from build123d import *

# Parameters (mm, degrees)
BOSS_EXTRUDE1_START = -169
SKETCH1_R           = 8
BOSS_EXTRUDE1_DEPTH = 294
SKETCH3_R           = 8
BOSS_EXTRUDE2_START = 159
SKETCH4_W           = 5.5
SKETCH4_H           = 3
BOSS_EXTRUDE2_DEPTH = 13
SKETCH5_W           = 11
SKETCH5_H           = 2


with BuildPart() as part:
    # Sketch1 → Boss-Extrude1 (new body)
    with BuildSketch(Plane(origin=(0, 0, 0), x_dir=(1, 0, 0), z_dir=(0, 1, 0)).offset(BOSS_EXTRUDE1_START)):
        with Locations(Location((0, 0, 0), (0, 0, 270))):
            Circle(SKETCH1_R)
    extrude(amount=BOSS_EXTRUDE1_DEPTH)

    # Sweep1: sweep along a path in Sketch2
    with BuildLine(Plane.XY) as sweep1_path:
        Line((-112, 176), (-51, 176))
        ThreePointArc((-51, 176), (-14.937554159, 161.062445841), (0, 125))
    # Sketch3 → Sweep1 (sweep)
    with BuildSketch(Plane(origin=(0, 125, 0), x_dir=(1, 0, 0), z_dir=(0, 1, 0))):
        Circle(SKETCH3_R)
    sweep(path=sweep1_path.line)

    # Sketch4 → Boss-Extrude2 (add)
    with BuildSketch(Plane(origin=(0, 0, 0), x_dir=(1, 0, 0), z_dir=(0, 1, 0)).offset(BOSS_EXTRUDE2_START)):
        with Locations((-106.25, 0)):
            Rectangle(SKETCH4_W, SKETCH4_H)
    extrude(amount=BOSS_EXTRUDE2_DEPTH)

    # Sketch5 → Revolve1 (revolve)
    with BuildSketch(Plane.XY, mode=Mode.PRIVATE) as revolve1_sk:
        with Locations((-103.5, 164)):
            Rectangle(SKETCH5_W, SKETCH5_H)
    revolve(revolve1_sk.sketch.rotate(Axis((-109, 163, 0), (1, 0, 0)), 90), axis=Axis((-109, 163, 0), (1, 0, 0)))


solid = part.part
Read the model definition and answer for the solid it produces. Units are mm, in the model's axes. A direction names the side the tool comes from. Give positions to 0.01 mm unless a question says otherwise; leave off trailing zeros. Write each loop counter-clockwise with the first axis right and the second up, starting at its lowest first coordinate (ties: lowest second). Pieces come first, ordered by that corner, then holes. Notation, with made-up numbers: M -32,87.25 L -4,87.25 A18 cw -4,100.25 Z; hole C 42,37 d9. An arc over 180 degrees is marked long. One line per item, written item: value. Start each with the question number.
(1) Find section A-A (z = 5.25). Determine the outline of the cut face in (x, y), plus the area to 3 significant figures.
(2) Find section C-C (x = -82.5). Determine the outline of the cut face in (y, z).
(3) Find section B-B (y = 67). Determine the outline of the cut face in (x, z).
(4) A tool of negligible diameter and unlimited length cuts with its end or side. For faces 1 (the flat face through (0, -169, 0)), 2 (the cylindrical face through (-7.81, -24.06, -1.73)), from which of +Z, -Z, +X, -X, +Y, -Y can it reach the whole face along a straight path? Write none if from no direction.
(5) Find the intervals of material crossed by line 1 (X direction, y = -76.5, z = 0); line 2 (Y direction, x = -50, z = -0.5); line 3 (Y direction, x = -80, z = -5) (3 decimals), in increasing order.
(6) Flat-ended cylindrical pins translate along their axes: pin 1 Ø2 at (y, z) = (162.5, 0) entering from +X; pin 2 Ø4 at (y, z) = (104, 4) entering from -X; pin 3 Ø4 at (x, z) = (-58.5, -6) entering from -Y. Find the tip coordinate at first contact, or state that the pin passes through.
Results below:
1. outline: M -112,169.96 L -51,169.96 A44.96 cw -6.04,125 L -6.04,-169 L 6.04,-169 L 6.04,125 A57.04 ccw -51,182.04 L -112,182.04 Z
1. area: 5,250 mm^2
2. outline: C 176,0 d16
3. outline: C 0,0 d16
4. face 1: +Z, -Z, +X, -X, -Y
4. face 2: -Y
5. line 1: x = -8 to 8
5. line 2: y = 168 to 183.98
5. line 3: y = 169.755 to 182.245
6. pin 1: stops at x = -4.65
6. pin 2: stops at x = -7.75
6. pin 3: stops at y = 169.07
